Here's how the part is built. I have some questions about the finished solid (model axes, mm). Give positions to 0.01 mm unless a question says otherwise; leave off trailing zeros. Loops run counter-clockwise (first coordinate to the right, second up) from the corner with the lowest first, then second, coordinate; pieces in that order, holes last.
Q1. Suppose I cut it at B-B (x = 164.5). List the corners of the cut face in (y, z) for me, and give its area (3 significant figures).
Q2. Suppose I cut it at A-A (z = 2.05). List the corners of the cut face in (x, y) for me.
Q3. Suppose I cut it at C-C (y = 603). List the corners of the cut face in (x, z) for me.
Q4. I need wall thicknesses on probe 1 along Y at (x, z) = (75, 1.7); probe 2 along X at (y, z) = (580, 1.1); probe 3 along Y at (x, z) = (260.5, 1.1). Which ranges of each line are inside material? Lowest first, please.
Autodesk Inventor part; units mm, degrees
ref_plane "YZ Plane" through (0, 0, 0) normal (1, 0, 0) x (0, 1, 0)
ref_plane "XZ Plane" through (0, 0, 0) normal (0, 1, 0) x (-1, 0, 0)
ref_plane "XY Plane" through (0, 0, 0) normal (0, 0, 1) x (1, 0, 0)
sketch "Esboço1" plane through (0, 0, 0) normal (0, 0, 1) x (1, 0, 0)
  line L0 (0, 0) -> (600, 0)
  line L1 (600, 0) -> (600, 700)
  line L2 (600, 700) -> (0, 700)
  line L3 (0, 700) -> (0, 0)
  dimension "d0" = 600
  dimension "d1" = 700
extrude "Extrusão1" add sketch "Esboço1" along normal blind 3
sketch "Esboço2" plane through (0, 0, 3) normal (0, 0, 1) x (1, 0, 0)
  line L0 (80, 620) -> (520, 620)
  line L1 (520, 620) -> (520, 180)
  line L2 (520, 180) -> (80, 180)
  line L3 (80, 180) -> (80, 620)
  line L4 (0, 700) -> (0, 0)
  line L5 (600, 0) -> (600, 700)
  line L6 (600, 700) -> (0, 700)
  line L7 (0, 0) -> (600, 0)
  dimension "d4" = 80
  dimension "d5" = 80
  dimension "d6" = 80
  dimension "d7" = 180
extrude "Extrusão2" cut sketch "Esboço2" against normal blind 10 contours L0 L1 L2 L3
fillet "Arredondamento1" radius 2 4 edges at (80, 620, 1.5) (520, 620, 1.5) (520, 180, 1.5) (80, 180, 1.5)
sketch "Esboço3" plane through (0, 0, 0) normal (0, 0, -1) x (-1, 0, 0)
  point P0 (0, 0)
  point P1 (-75, 220)
  point P2 (-75, 227)
  point P3 (-75, 580)
  point P4 (-75, 573)
hole "Furo1" at (75, 220, 0) at (75, 227, 0) at (75, 580, 0) at (75, 573, 0) direction (0, 0, 1) diameter 2 end through all
sketch "Esboço4" plane through (0, 0, 0) normal (0, 0, -1) x (-1, 0, 0)
  line L0 (-80, 618) -> (-80, 182)
  line L1 (-80, 232.8077) -> (-77, 232.8077)
  line L2 (-77, 232.8077) -> (-77, 214.8077)
  line L3 (-77, 214.8077) -> (-80, 214.8077)
  line L4 (-80, 214.8077) -> (-80, 232.8077)
  line L5 (-80, 586.0371) -> (-77, 586.0371)
  line L6 (-77, 586.0371) -> (-77, 568.0371)
  line L7 (-77, 568.0371) -> (-80, 568.0371)
  line L8 (-80, 568.0371) -> (-80, 586.0371)
  point P0 (0, 0)
  point P1 (-80, 586.0371)
  dimension "d19" = 3
  dimension "d20" = 18
  dimension "d21" = 3
  dimension "d22" = 18
extrude "Extrusão3" cut sketch "Esboço4" against normal blind 10
properties part number "frente" material "MDF - Chapa de fibra de média densidade"
Solutions:
1. outline: (0, 0) - (180, 0) - (180, 3) - (0, 3) - close; (620, 0) - (700, 0) - (700, 3) - (620, 3) - close
1. area: 780 mm2
2. outline: (0, 0) - (600, 0) - (600, 700) - (0, 700) - close; hole circle Ø2 at (75, 220); hole circle Ø2 at (75, 227); hole circle Ø2 at (75, 573); hole circle Ø2 at (75, 580); hole (77, 214.81) - (80, 214.81) - (80, 182) arc R2 ccw to (82, 180) - (518, 180) arc R2 ccw to (520, 182) - (520, 618) arc R2 ccw to (518, 620) - (82, 620) arc R2 ccw to (80, 618) - (80, 586.04) - (77, 586.04) - (77, 568.04) - (80, 568.04) - (80, 232.81) - (77, 232.81) - close
3. outline: (0, 0) - (80, 0) - (80, 3) - (0, 3) - close; (520, 0) - (600, 0) - (600, 3) - (520, 3) - close
4. probe 1: y = 0 to 219, 221 to 226, 228 to 572, 574 to 579, 581 to 700
4. probe 2: x = 0 to 74, 76 to 77, 520 to 600
4. probe 3: y = 0 to 180, 620 to 700
